Part model, mm, in its own coordinate system. A direction names the side the tool comes from. Round coordinates to 2 decimals unless told otherwise and drop trailing zeros. Order: outer loops, then holes, each group sorted by start corner. A loop starts at its lowest first (then second) coordinate and runs counter-clockwise, first axis right, second up. Notation, with made-up numbers: (49, 1) -> (101, 1) arc R9 cw to (101, 14) -> close; hole circle Ø4 at (15.25, 75.25). An arc over 180 degrees is marked (long way). Answer as a JSON object with one key per item and string values. Group by question number.
Autodesk Inventor part; units mm, degrees
ref_plane "YZ Plane" through (0, 0, 0) normal (1, 0, 0) x (0, 1, 0)
ref_plane "XZ Plane" through (0, 0, 0) normal (0, 1, 0) x (-1, 0, 0)
ref_plane "XY Plane" through (0, 0, 0) normal (0, 0, 1) x (1, 0, 0)
sketch "Sketch1" plane through (0, 0, 0) normal (0, 0, 1) x (1, 0, 0)
  line L0 (-12.7, -12.7) -> (12.7, -12.7)
  line L1 (12.7, -12.7) -> (12.7, 12.7)
  line L2 (12.7, 12.7) -> (-12.7, 12.7)
  line L3 (-12.7, 12.7) -> (-12.7, -12.7)
  line L4 (-12.7, -12.7) -> (12.7, 12.7) construction
  line L5 (12.7, -12.7) -> (-12.7, 12.7) construction
  line L6 (-9.525, -9.525) -> (9.525, -9.525)
  line L7 (9.525, -9.525) -> (9.525, 9.525)
  line L8 (9.525, 9.525) -> (-9.525, 9.525)
  line L9 (-9.525, 9.525) -> (-9.525, -9.525)
  line L10 (-9.525, -9.525) -> (9.525, 9.525) construction
  line L11 (9.525, -9.525) -> (-9.525, 9.525) construction
  point P0 (0, 0)
  dimension "d0" = 25.4
  dimension "d1" = 25.4
  dimension "d2" = 3.175
  dimension "d3" = 3.175
extrude "Extrusion1" add sketch "Sketch1" along normal mid plane 73.025
properties part number "2_875-inchAluminumTubing" material "Aluminum 6061"
Q1. Band-saw the part on A-A (x = -7.25). List the corners of the cut face in (y, z) (1 decimal).
Q2. Two-plate mould, pull along X, no slides. Class faces 3 (the flat face through (0, -9.525, -1)), 4 (the flat face through (-12.7, 0, -1)), 5 (the flat face through (11, 0, 36.512)): +X half, -X half, draft (parallel to the pull), parting line (faces both ways), or undercut.
Q3. Wall check: line 1 (Y direction, x = -7.75, z = 25.5) (3 decimals). Give the ranges that are in metal, low to high. Write a range as [from, to].
Q4. Band-saw the part on C-C (z = 23.5). List the corners of the cut face in (x, y) (3 decimals), plus the area to 3 significant figures.
Q5. Which spindle directions (+Z, -Z, +X, -X, +Y, -Y) get a long thin tool onto all of the face, cutting with end or side? Do faces 1 (the flat face through (11, 0, -36.512)), 2 (the flat face through (0, 9.525, -1)). Say none if no direction does.
Completed:
{
 "1": {"outline": "(-12.7, -36.5) -> (-9.5, -36.5) -> (-9.5, 36.5) -> (-12.7, 36.5) -> close; (9.5, -36.5) -> (12.7, -36.5) -> (12.7, 36.5) -> (9.5, 36.5) -> close"},
 "2": {"face 3": "undercut", "face 4": "-X half", "face 5": "draft"},
 "3": {"line 1": "[-12.7, -9.525], [9.525, 12.7]"},
 "4": {"outline": "(-12.7, -12.7) -> (12.7, -12.7) -> (12.7, 12.7) -> (-12.7, 12.7) -> close; hole (-9.525, -9.525) -> (9.525, -9.525) -> (9.525, 9.525) -> (-9.525, 9.525) -> close", "area": "282 mm2"},
 "5": {"face 1": "-Z, +X, -X, +Y, -Y", "face 2": "+Z, -Z"}
}
